Geometry: see drawing. Coordinates: mm, zero at the bounding-box minimum. A direction names the side the tool comes from. Give positions to 0.01 mm unless a question says otherwise; leave off trailing zeros. Write each loop counter-clockwise with the first axis right and the second up, starting at its lowest first coordinate (ties: lowest second). Pieces come first, ordered by that corner, then holes. Notation, with made-up numbers: (-16.5, -4.5) -> (33.5, -4.5) arc R22 ccw to (33.5, 11.5) -> close; hole circle Ø2 at (74.25, 19.5). An arc over 180 degrees is marked (long way). Write item = value, one per line.
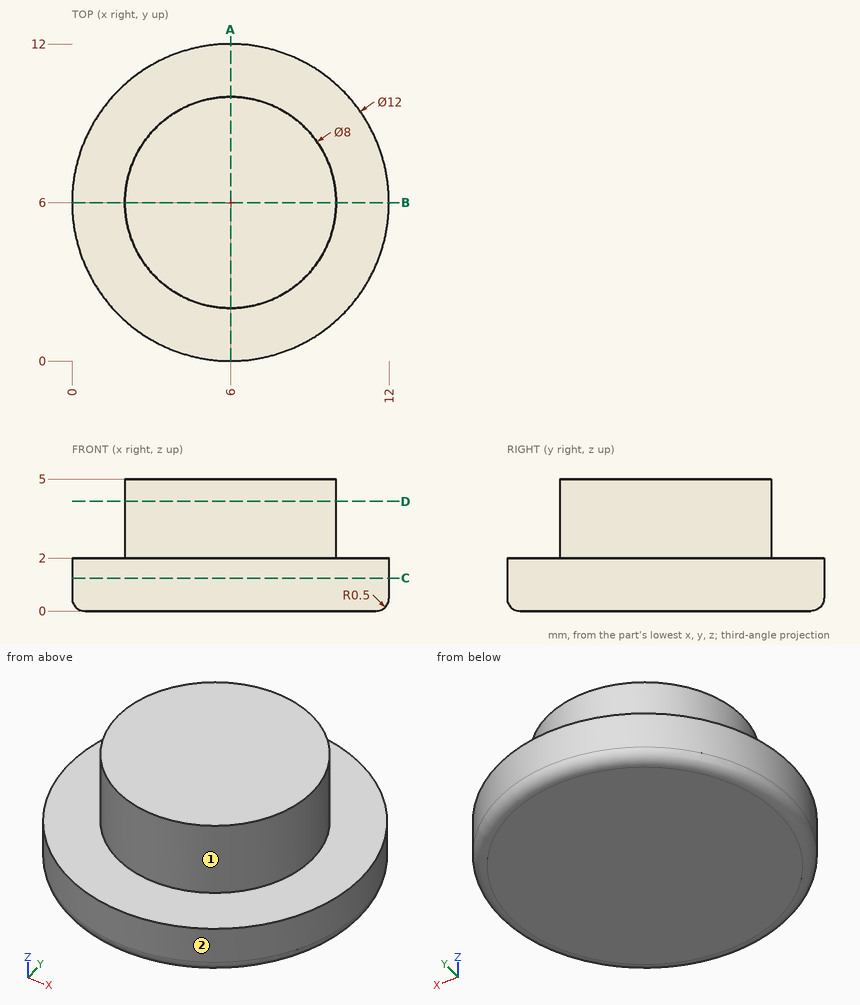
(1) Section query C-C (z = 1.25). Return loops of the section in (x, y), plus the area to 3 significant figures.
Values follow:
outline = circle Ø12 at (6, 6)
area = 113 mm2
(2) Material intervals for line 1 (Z direction, x = 2.25, y = 8); line 2 (X direction, y = 9.25, z = 2.5); line 3 (X direction, y = 6.5, z = 3.8), sorted ascending.
Values follow:
line_1 = 0 to 2
line_2 = 3.67 to 8.33
line_3 = 2.03 to 9.97
(3) First-contact query: pin 1 (1 mm diameter, centred on x = 1.5, z = 2, fed in from +Y); pin 2 (1.5 mm diameter, centred on x = 6.5, z = 4.5, fed in from -Y). Flat tips, straight axial feed; report the tip coordinate or a pass-through.
Values follow:
pin_1 = 10.47
pin_2 = 2
(4) Section query A-A (x = 6). Return loops of the section in (y, z).
Values follow:
outline = (0, 0.5) arc R0.5 ccw to (0.5, 0) -> (11.5, 0) arc R0.5 ccw to (12, 0.5) -> (12, 2) -> (10, 2) -> (10, 5) -> (2, 5) -> (2, 2) -> (0, 2) -> close
(5) Section query D-D (z = 4.15). Return loops of the section in (x, y), plus the area to 3 significant figures.
Values follow:
outline = circle Ø8 at (6, 6)
area = 50.3 mm2
(6) Access query for the marked faces 1 and 2. Directions: +Z, -Z, +X, -X, +Y, -Y. A direction counts if a zero-diameter tool reaches every point of the face in a straight line with its end or side. Return the directions, or none.
Values follow:
face_1 = +Z
face_2 = +Z, -Z
